Model file for the job. Use its own axes, mm. Coordinates: 2 decimals unless noted, no trailing zeros. Order: outer loops, then holes, each group sorted by start corner. A loop starts at its lowest first (then second) coordinate and runs counter-clockwise, first axis right, second up. Notation, with made-up numbers: (66.25, -5) -> (70.25, -5) arc R34 ccw to (70.25, 31) -> close; hole circle Ø9 at (85, -28). An arc over 180 degrees is marked (long way). Return JSON: item names as keys, results as strings. Group by question number.
1) Cut at A-A (x = -34.5). Write the cut outline in (y, z), and give its area (3 significant figures).
2) Cut at C-C (x = 43). Write the cut outline in (y, z).
3) Probe line 1 (X direction, y = 2.7, z = -20); line 2 (X direction, y = 2.95, z = -3.25); line 3 (X direction, y = 2.1, z = -11.75). List the from-to ranges inside material, lowest first.
4) Cut at D-D (z = -9.5). Write the cut outline in (x, y), and give its area (3 significant figures).
5) Cut at B-B (z = -5.5). Write the cut outline in (x, y).
6) Flat gauge pins, fed straight in: pin 1 (2 mm diameter, centred on x = -10, z = -11, fed in from -Y); pin 2 (1 mm diameter, centred on y = 2, z = -11, fed in from -X); pin 3 (2 mm diameter, centred on y = 2, z = -9.5, fed in from -X); pin 4 (0.8 mm diameter, centred on y = 2, z = -1, fed in from +X). Where does each tip first touch, or does it go through?
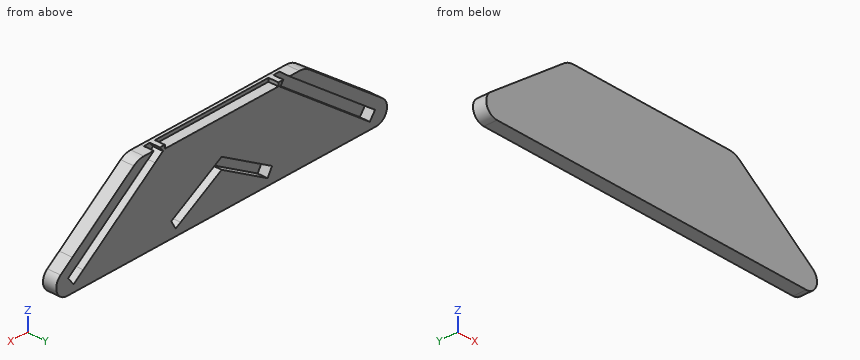
Autodesk Fusion 360 part; units mm, degrees
sketch "Sketch1" plane through (0, 0, 0) normal (0, 1, 0) x (1, 0, 0)
  line L0 (0, 0) -> (0, 239.8445)
  line L1 (0, 0) -> (0, 25)
  line L2 (0, 0) -> (-94.6434, 191.0764)
  line L3 (0, 0) -> (0, 15.4)
  line L4 (-10.6829, 21.5678) -> (-95.942, 70.7921)
  line L5 (13.3368, 23.1) -> (-199.4619, 9.5254)
  line L6 (-26.6736, 0) -> (-59.8805, 24.6504)
  line L7 (-33.0314, -39.3634) -> (-81.6324, 168.2553)
  line L8 (-33.0314, -39.3634) -> (21.6354, 194.1681)
  line L9 (-33.0314, -39.3634) -> (0, -39.3634)
  line L10 (-22.0861, 0.9535) -> (-23.3706, 1.907)
  line L11 (-49.9408, 21.6308) -> (-57.7944, 27.4607)
  line L12 (-23.3706, 1.907) -> (-46.756, 19.2666)
  line L13 (0, 15.4) -> (-10.6829, 21.5678)
  line L14 (-10.6829, 21.5678) -> (-14.9643, 24.0396)
  line L15 (0, 11.9359) -> (-12.1829, 18.9697)
  line L16 (-12.1829, 18.9697) -> (-16.4643, 21.4416)
  line L17 (-16.4643, 21.4416) -> (-14.9643, 24.0396)
  line L18 (-14.9643, 24.0396) -> (-59.0578, 24.0396)
  line L19 (-20.0907, 0.9577) -> (-19.0135, 2.4088)
  line L20 (-48.1526, 24.0396) -> (-49.9408, 21.6308)
  line L21 (-19.0135, 2.4088) -> (-21.5824, 4.3158)
  line L22 (-21.5824, 4.3158) -> (-44.9679, 21.6755)
  line L23 (-44.9679, 21.6755) -> (-48.1526, 24.0396)
  line L24 (-57.7944, 27.4607) -> (-56.0062, 29.8696)
  line L25 (-46.756, 19.2666) -> (-49.9408, 21.6308)
  line L26 (-48.1526, 24.0396) -> (-56.0062, 29.8696)
  line L27 (0, 0) -> (0, 1)
  line L28 (0, 1) -> (-20.0907, 0.9577)
  line L29 (13.3368, 23.1) -> (-20.5394, 3.5416)
  line L30 (-23.3706, 1.907) -> (-194.3746, -96.8223)
  line L31 (-20.5394, 3.5416) -> (-23.3706, 1.907)
  line L32 (-22.0861, 0.9535) -> (-20.298, 3.3623)
  line L33 (-20.0907, 0.9577) -> (-22.0861, 0.9535)
  line L34 (0, 0) -> (0, 25)
  line L35 (0, 1) -> (0, 2)
  line L36 (0, 2) -> (-19.317, 2)
  line L37 (-19.317, 2) -> (-19.3148, 0.9593)
  line L38 (46.756, 19.2666) -> (49.9408, 21.6308)
  line L39 (48.1526, 24.0396) -> (49.9408, 21.6308)
  line L40 (44.9679, 21.6755) -> (48.1526, 24.0396)
  line L41 (21.5824, 4.3158) -> (44.9679, 21.6755)
  line L42 (23.3706, 1.907) -> (46.756, 19.2666)
  line L43 (22.0861, 0.9535) -> (23.3706, 1.907)
  line L44 (20.0907, 0.9577) -> (19.0135, 2.4088)
  line L45 (19.0135, 2.4088) -> (21.5824, 4.3158)
  line L46 (20.0907, 0.9577) -> (22.0861, 0.9535)
  line L47 (0, 11.9359) -> (12.1829, 18.9697)
  line L48 (16.4643, 21.4416) -> (14.9643, 24.0396)
  line L49 (12.1829, 18.9697) -> (16.4643, 21.4416)
  line L50 (10.6829, 21.5678) -> (14.9643, 24.0396)
  line L51 (0, 15.4) -> (10.6829, 21.5678)
  line L52 (0, 1) -> (20.0907, 0.9577)
  line L53 (14.9643, 24.0396) -> (59.0578, 24.0396)
  line L54 (0, 2) -> (19.317, 2)
  line L55 (19.317, 2) -> (19.3148, 0.9593)
  line L56 (-14.9643, 24.0396) -> (14.9643, 24.0396)
  line L57 (0, 1) -> (35.9633, 0.9243)
  line L58 (0, 1) -> (-40.1034, 0.9577)
  line L59 (-23.8743, -1.4553) -> (-25.1587, -0.5018)
  line L60 (-25.1587, -0.5018) -> (-48.5442, 16.8578)
  line L61 (-48.5442, 16.8578) -> (-51.7289, 19.2219)
  line L62 (-51.7289, 19.2219) -> (-60.9132, 26.0396)
  line L63 (-14.9643, 26.0396) -> (-60.9132, 26.0396)
  line L64 (-14.9643, 26.0396) -> (14.9643, 26.0396)
  line L65 (14.9643, 26.0396) -> (60.9132, 26.0396)
  line L66 (23.8743, -1.4553) -> (25.1587, -0.5018)
  line L67 (25.1587, -0.5018) -> (48.5442, 16.8578)
  line L68 (28.529, 2) -> (60.9132, 26.0396)
  line L69 (18.4918, 0.9611) -> (18.4918, 2)
  line L70 (-18.5464, 0.9609) -> (-18.5464, 2)
  line L71 (19.1327, 2.2483) -> (21.7016, 4.1552)
  line L72 (21.7016, 4.1552) -> (45.0871, 21.5149)
  line L73 (45.0871, 21.5149) -> (48.2719, 23.879)
  line L74 (-0.1, 12.1091) -> (12.0829, 19.1429)
  line L75 (12.0829, 19.1429) -> (16.3643, 21.6148)
  line L76 (-0.05, 12.0225) -> (12.1329, 19.0563)
  line L77 (12.1329, 19.0563) -> (16.4143, 21.5282)
  line L78 (19.0731, 2.3285) -> (21.642, 4.2355)
  line L79 (21.642, 4.2355) -> (45.0275, 21.5952)
  line L80 (45.0275, 21.5952) -> (48.2123, 23.9593)
  dimension "d9" = 25
  dimension "d11" = 15.4
  dimension "d21" = 1
  dimension "d37" = 0.2
  dimension "d38" = 0.2
  dimension "d39" = 0.1
  dimension "d40" = 0.1
extrude "Extrude2" add sketch "Sketch1" along normal blind 1 contours L0 L1 L3 L34 L35 L52 L54 L57 L69 | L0 L1 L3 L34 L40 L41 L44 L45 L47 L48 L49 L53 L54 | L52 L54 L55 L57 L69 | L0 L1 L3 L34 L47 L48 L49 L76 L77 | L44 L52 L55 L57 | L0 L1 L3 L34 L48 L74 L75 L76 L77 | L38 L39 L42 L43 L44 L46 L57 L71 L72 L73 | L0 L1 L3 L29 L34 L48 L50 L51 L74 L75 | L0 L1 L5 L29 L34 L50 L51 | L39 L44 L71 L72 L73 L78 L79 L80 | L38 L39 L42 L43 L53 L57 L67 L68 | L0 L1 L5 L34 L50 L56 | L39 L40 L41 L44 L45 L78 L79 L80 | L0 L1 L34 L53 L56 L64 L65 L68 makes body 1
extrude "Extrude3" add sketch "Sketch1" along normal blind 4 separate body contours L0 L1 L3 L34 L40 L41 L44 L45 L47 L48 L49 L53 L54 | L52 L54 L55 L57 L69 | L0 L1 L3 L34 L47 L48 L49 L76 L77 | L44 L52 L55 L57 | L0 L1 L5 L29 L34 L50 L51 | L38 L39 L42 L43 L53 L57 L67 L68 | L0 L1 L5 L34 L50 L56 | L39 L40 L41 L44 L45 L78 L79 L80 | L0 L1 L34 L53 L56 L64 L65 L68 makes body 2
mirror "Mirror1" about plane through (0, 0, 0) normal (1, 0, 0) of bodies 2 1 makes body 3 at (-27.8999, 0, -15.9387) makes body 4 at (-29.3394, 1, -17.6741)
combine "Combine1" operation add target body 4 tool bodies 3 2 1
fillet "Fillet2" radius 3.5 1 edges at (60.9132, 2, -26.0396) on bodies 4
fillet "Fillet3" radius 5.5 1 edges at (27.105, 2, -0.9429) on bodies 4
fillet "Fillet4" radius 5.5 1 edges at (-27.105, 2, -0.9429) on bodies 4
fillet "Fillet5" radius 3.5 1 edges at (-60.9132, 2, -26.0396) on bodies 4
equation "AA = 1.1 mm"
Answers below:
{
 "1": {"outline": "(0, -26.04) -> (4, -26.04) -> (4, -13.78) -> (1, -13.78) -> (1, -10.17) -> (4, -10.17) -> (4, -6.43) -> (0, -6.43) -> close", "area": "67.6 mm^2"},
 "2": {"outline": "(0, -26.04) -> (4, -26.04) -> (4, -20.09) -> (1, -20.09) -> (1, -16.48) -> (4, -16.48) -> (4, -12.74) -> (0, -12.74) -> close"},
 "3": {"line 1": "x = -52.73 to -47.74, -42.88 to -13.77, -7.97 to 7.97, 13.77 to 42.88, 47.74 to 52.73", "line 2": "x = -30.21 to -25.18, -20.31 to 20.31, 25.18 to 30.21", "line 3": "x = -41.66 to -36.63, -31.76 to 31.76, 36.63 to 41.66"},
 "4": {"outline": "(-38.63, 0) -> (38.63, 0) -> (38.63, 4) -> (33.6, 4) -> (33.6, 1) -> (28.73, 1) -> (28.73, 4) -> (-28.73, 4) -> (-28.73, 1) -> (-33.6, 1) -> (-33.6, 4) -> (-38.63, 4) -> close", "area": "280 mm^2"},
 "5": {"outline": "(-33.24, 0) -> (33.24, 0) -> (33.24, 4) -> (28.21, 4) -> (28.21, 1) -> (23.35, 1) -> (23.35, 4) -> (-23.35, 4) -> (-23.35, 1) -> (-28.21, 1) -> (-28.21, 4) -> (-33.24, 4) -> close"},
 "6": {"pin 1": "stops at y = 0", "pin 2": "stops at x = -41.33", "pin 3": "stops at x = -39.98", "pin 4": "stops at x = 27.48"}
}
